Autodesk Inventor part; units mm, degrees
ref_plane "YZ Plane" through (0, 0, 0) normal (1, 0, 0) x (0, 1, 0)
ref_plane "XZ Plane" through (0, 0, 0) normal (0, 1, 0) x (-1, 0, 0)
ref_plane "XY Plane" through (0, 0, 0) normal (0, 0, 1) x (1, 0, 0)
sketch "Sketch1" plane through (0, 0, 0) normal (0, 0, 1) x (1, 0, 0)
  line L0 (4, 9.5) -> (4, 4) construction
  line L1 (0.75, 6.75) -> (0.75, 13.5)
  line L2 (0.75, 13.5) -> (7.25, 13.5)
  line L3 (7.25, 13.5) -> (7.25, 6.75)
  line L4 (0, 6.75) -> (0, 0)
  line L5 (0, 0) -> (8, 0)
  line L6 (8, 0) -> (8, 6.75)
  line L7 (0, 6.75) -> (0.75, 6.75)
  line L8 (7.25, 6.75) -> (8, 6.75)
  line L9 (0.75, 6.75) -> (7.25, 6.75) construction
  line L10 (4, 4) -> (4, 0) construction
  line L11 (4, 9.5) -> (4, 13.5) construction
  line L12 (3.25, 12.125) -> (4.75, 12.125)
  line L13 (4.75, 12.125) -> (4.75, 8.125)
  line L14 (4.75, 8.125) -> (3.25, 8.125)
  line L15 (3.25, 8.125) -> (3.25, 12.125)
  line L16 (2, 4.125) -> (6, 4.125)
  line L17 (6, 4.125) -> (6, 2.625)
  line L18 (6, 2.625) -> (2, 2.625)
  line L19 (2, 2.625) -> (2, 4.125)
  line L20 (4.75, 12.125) -> (4.75, 13.5) construction
  line L21 (4.75, 8.125) -> (4.75, 6.75) construction
  line L22 (6, 2.625) -> (6, 0) construction
  line L23 (6, 4.125) -> (6, 6.75) construction
  point P0 (4, 6.75)
  dimension "d2" = 5.5
  dimension "d3" = 6.5
  dimension "d4" = 8
  dimension "d5" = 13.5
  dimension "d9" = 1.5
  dimension "d10" = 4
  dimension "d11" = 4
  dimension "d12" = 1.5
extrude "Extrusion2" add sketch "Sketch1" along normal blind 6
fillet "Fillet2" radius 0.5 8 edges at (7.25, 6.75, 3) (8, 6.75, 3) (0, 6.75, 3) (0.75, 6.75, 3) (0, 0, 3) (8, 0, 3) (7.25, 13.5, 3) (0.75, 13.5, 3)
extrude "Extrusion3" add sketch "Sketch1" along normal blind 12.5 contours L12 L13 L14 L15 | L16 L17 L18 L19
sketch "Sketch2" plane through (0, 0, 0) normal (0, 0, -1) x (-1, 0, 0)
  line L0 (-6, 4.125) -> (-2, 4.125) construction
  line L1 (-2, 4.125) -> (-2, 2.625) construction
  line L2 (-2, 2.625) -> (-6, 2.625) construction
  line L3 (-6, 2.625) -> (-6, 4.125) construction
  line L4 (-4.75, 12.125) -> (-3.25, 12.125) construction
  line L5 (-3.25, 12.125) -> (-3.25, 8.125) construction
  line L6 (-3.25, 8.125) -> (-4.75, 8.125) construction
  line L7 (-4.75, 8.125) -> (-4.75, 12.125) construction
  line L8 (-3.25, 8.125) -> (-3.25, 12.125) construction
  line L9 (-3.25, 12.125) -> (-4.75, 8.125) construction
  line L10 (-3.25, 12.125) -> (-4.75, 12.125) construction
  line L11 (-3.25, 8.125) -> (-4.75, 12.125) construction
  line L12 (-2, 4.125) -> (-6, 2.625) construction
  line L13 (-6, 2.625) -> (-2, 2.625) construction
  line L14 (-6, 2.625) -> (-6, 4.125) construction
  line L15 (-2, 2.625) -> (-6, 4.125) construction
  circle A0 centre (-4, 10.125) radius 1.75
  circle A1 centre (-4, 3.375) radius 1.75
  point P0 (0, 0)
  dimension "d18" = 3.5
  dimension "d19" = 3.5
extrude "Extrusion4" add sketch "Sketch2" along normal blind 4
fillet "Fillet3" radius 0.5 4 edges at (4, 12.125, 12.5) (4, 8.125, 12.5) (2, 3.375, 12.5) (6, 3.375, 12.5)
properties part number "Tplug"
Design review of the part built by this model. Coordinates are the model's own, in mm. A direction names the side the tool comes from. Round coordinates to 2 decimals unless told otherwise and drop trailing zeros. Loops run counter-clockwise (first coordinate to the right, second up) from the corner with the lowest first, then second, coordinate; pieces in that order, holes last. Notation, with made-up numbers: (-20.75, -33) -> (38.25, -33) arc R24 ccw to (38.25, -21) -> close; hole circle Ø9 at (-23.5, -18.75). An arc over 180 degrees is marked (long way). Use one line per item in the form item = value. Start each with the question number.
Q1. We need section C-C on y = 3. Give the boundary of the cut face in (x, z), then the cut area to 3 significant figures.
Q2. Machinability: for faces 1 (the face through (4, 12.125, 9)), 2 (the face through (2, 3, 9)), 3 (the face through (5.29, 8.94, -1.97)), 4 (the face through (0.75, 10, 3)), which of the approach directions +Z, -Z, +X, -X, +Y, -Y give a long, thin tool a straight path to every point of the face, cutting with its end or side? Answer none if there is none.
Q3. Draft analysis for pull direction Y (two halves, no side actions). For faces 5 (the face through (7.25, 10, 3)), 6 (the face through (4, 13.5, 3)), 7 (the face through (4, 7, 0)), state which applies: +Y half, -Y half, draft (parallel to the pull), parting line (faces both ways), or undercut.
Q4. For pin 1 Ø3 at (y, z) = (9.5, 7) entering from +X; pin 2 Ø1.2 at (y, z) = (3.5, 9.5) entering from +X; pin 3 Ø4.5 at (x, z) = (4, 8.5) entering from +Y (3 decimals), all flat-tipped, find the tip position at first contact; note any pin that passes through.
Q5. We need section D-D on y = 1.25. Give the boundary of the cut face in (x, z).
Q6. We need section A-A on z = 8.25. Give the boundary of the cut face in (x, y) (3 decimals).
Q7. Wall thickness on line 1 along X through (y, z) = (9.25, 4.25); line 2 along Z through (x, y) = (6.75, 6); line 3 along X through (y, z) = (9, 9.75): over which ranges is each line inside the solid? List them lowest first. Write a range as [from, to].
Q8. We need section B-B on x = 4. Give the boundary of the cut face in (y, z) (3 decimals), then the cut area to 3 significant figures.
Calculated:
q1.outline = (0, 0) -> (2.29, 0) -> (2.29, -4) -> (5.71, -4) -> (5.71, 0) -> (8, 0) -> (8, 6) -> (6, 6) -> (6, 12) arc R0.5 ccw to (5.5, 12.5) -> (2.5, 12.5) arc R0.5 ccw to (2, 12) -> (2, 6) -> (0, 6) -> close
q1.area = 87.6 mm²
q2.face_1 = +Z, +X, -X, +Y
q2.face_2 = +Z, -X, +Y, -Y
q2.face_3 = -Z
q2.face_4 = +Z, -Z, -X, +Y
q3.face_5 = draft
q3.face_6 = +Y half
q3.face_7 = undercut
q4.pin_1 = 7.25
q4.pin_2 = 6
q4.pin_3 = 12.125
q5.outline = (0, 0) -> (8, 0) -> (8, 6) -> (0, 6) -> close
q6.outline = (2, 2.625) -> (6, 2.625) -> (6, 4.125) -> (2, 4.125) -> close; (3.25, 8.125) -> (4.75, 8.125) -> (4.75, 12.125) -> (3.25, 12.125) -> close
q7.line_1 = [0.75, 7.25]
q7.line_2 = [0, 6]
q7.line_3 = [3.25, 4.75]
q8.outline = (0, 0) -> (1.625, 0) -> (1.625, -4) -> (5.125, -4) -> (5.125, 0) -> (8.375, 0) -> (8.375, -4) -> (11.875, -4) -> (11.875, 0) -> (13.5, 0) -> (13.5, 6) -> (12.125, 6) -> (12.125, 12) arc R0.5 ccw to (11.625, 12.5) -> (8.625, 12.5) arc R0.5 ccw to (8.125, 12) -> (8.125, 6) -> (4.125, 6) -> (4.125, 12.5) -> (2.625, 12.5) -> (2.625, 6) -> (0, 6) -> close
q8.area = 145 mm²
